Input: part model. Units: mm. Frame: model coordinates. A direction names the side the tool comes from. Round coordinates to 2 decimals unless told otherwise and drop trailing zeros. Write each loop counter-clockwise with the first axis right and the second up, starting at its lowest first coordinate (ties: lowest second). Pieces come first, ordered by that corner, then holes. Notation, with made-up numbers: M 18,82 L 27,82 A36 ccw 27,119 Z; hole C 34.25,9.25 d7. An arc over 180 degrees is marked long. Answer as CSV lines item,"result". Start each with the question number.
Autodesk Inventor part; units mm, degrees
ref_plane "YZ Plane" through (0, 0, 0) normal (1, 0, 0) x (0, 1, 0)
ref_plane "XZ Plane" through (0, 0, 0) normal (0, 1, 0) x (-1, 0, 0)
ref_plane "XY Plane" through (0, 0, 0) normal (0, 0, 1) x (1, 0, 0)
sketch "Sketch1" plane through (0, 0, 0) normal (0, 1, 0) x (-1, 0, 0)
  line L0 (0, 0) -> (6.2, 0)
  line L1 (6.2, 0) -> (6.2, 9.5)
  line L2 (6.2, 9.5) -> (0, 9.5)
  line L3 (0, 9.5) -> (0, 0)
  circle A0 centre (3.1, 0) radius 3.1
  circle A1 centre (3.1, 0) radius 1
  dimension "d2" = 6.2
  dimension "d3" = 9.5
  dimension "d4" = 2
extrude "Extrusion1" add sketch "Sketch1" along normal blind 3 contours A1 L0 A0 | L0 A0 A1 | A0 L3 L2 L1
sketch "Sketch2" plane through (0, 3, 0) normal (0, 1, 0) x (1, 0, 0)
  circle A0 centre (-3.1, 0) radius 1
  line L0 (-6.2, 0) -> (-6.2, -9.5)
  circle A1 centre (-3.1, 0) radius 3.1
  circle A2 centre (-3.1, 0) radius 1
  point P0 (0, 0)
extrude "Extrusion2" add sketch "Sketch2" along normal blind 12.5
sketch "Sketch3" plane through (0, 3, 0) normal (0, 1, 0) x (1, 0, 0)
  line L0 (-6.2, -9.5) -> (0, -9.5)
  line L1 (-6.2, -9.5) -> (0, -9.5)
  line L2 (0, -9.5) -> (0, -11.5)
  line L3 (0, -11.5) -> (-6.2, -11.5)
  line L4 (-6.2, -11.5) -> (-6.2, -9.5)
  point P0 (0, 0)
  dimension "d9" = 2
extrude "Extrusion3" add sketch "Sketch3" against normal blind 4
ref_plane "Work Plane1" through (-3.1, 0, 0) normal (1, 0, 0) x (0, 0, -1)
sketch "Sketch4" plane through (-3.1, 0, 0) normal (1, 0, 0) x (0, 0, -1)
  line L0 (-11.5, 3) -> (0, 3)
  line L1 (3.1, 15.5) -> (-3.1, 15.5)
  line L2 (-11.5, 3) -> (-3.1, 15.5)
  line L3 (-1, 15.5) -> (1, 15.5)
  line L4 (-3.1, 15.5) -> (-1, 15.5)
  line L5 (-1, 15.5) -> (-1, 3)
  line L6 (-11.5, 3) -> (-11.5, -1)
  line L7 (-1, 3) -> (-11.5, 3)
  point P0 (0, 0)
extrude "Extrusion4" add sketch "Sketch4" along normal mid plane 2
properties part number "Pi3B_spacer_F"
Item 1: Access query for faces 4 (the face through (-3.2, 7.6, -3.1)), 5 (the face through (-3, 0, 3)), 6 (the face through (-1, 3, 7)), 7 (the face through (-5, 3, 7)). Directions: +Z, -Z, +X, -X, +Y, -Y. A direction counts if a zero-diameter tool reaches every point of the face in a straight line with its end or side. Return the directions, or none.
Item 2: Cut plane D-D, the plane x = -0.25. Return loops of the section in (y, z), plus the area to 3 significant figures.
Item 3: Pin query (flat end, axial travel): pin 1 Ø1 at (x, z) = (-5.5, 6.5) entering from -Y; pin 2 Ø4.5 at (y, z) = (8.5, 6.5) entering from +X; pin 3 Ø1.7 at (x, z) = (-5.5, 5) entering from +Y. Return the tip coordinate at first contact, or that it passes through.
Item 4: Cut plane A-A, the plane y = 1.5. Return loops of the section in (x, z), plus the area to 3 significant figures.
Item 5: Draft query along Z for faces 1 (the face through (-3.034, 7.642, 0.998)), 2 (the face through (-3.1, -0.5, 9.5)), 3 (the face through (-4, 15.5, -1)). Return one class per face: +Z half, -Z half, draft (parallel to the pull), parting line (faces both ways), or undercut.
Item 6: Line query: line 1 (X direction, y = 9.75, z = 0); line 2 (Y direction, x = -4.5, z = 3.5); line 3 (X direction, y = 3.5, z = 7). Output: solid intervals per line, ascending. Write a range as [from, to].
Item 7: Cut plane B-B, the plane z = 10.75. Return loops of the section in (x, y).
Results list:
1,face 4,"+Y"
1,face 5,"-Z, +X, -X, -Y"
1,face 6,"+Z, +X, +Y"
1,face 7,"+Z, -X, +Y"
2,outline,"M -1,9.5 L 0,9.5 L 0,-1.22 L 15.5,-1.22 L 15.5,1.22 L 3,1.22 L 3,11.5 L -1,11.5 Z"
2,area,"70.6 mm²"
3,pin 1,"y = 0"
3,pin 2,"x = -2.1"
3,pin 3,"y = 3"
4,outline,"M -6.2,0 A3.1 ccw 0,0 L 0,11.5 L -6.2,11.5 Z; hole C -3.1,0 d2"
4,area,"83.3 mm²"
5,face 1,"undercut"
5,face 2,"-Z half"
5,face 3,"draft"
6,line 1,"[-6.2, -4.1], [-2.1, 0]"
6,line 2,"[0, 3]"
6,line 3,"[-4.1, -2.1]"
7,outline,"M -6.2,-1 L 0,-1 L 0,3 L -2.1,3 L -2.1,4.12 L -4.1,4.12 L -4.1,3 L -6.2,3 Z"
